Geometry: final body of the model. Coordinates: model frame, mm. A direction names the side the tool comes from. Give positions to 0.01 mm unless a question says otherwise; leave off trailing zeros. Order: outer loops, then holes, each group sorted by start corner. A loop starts at its lowest first (then second) coordinate and runs counter-clockwise, first axis right, second up. Notation, with made-up numbers: (-10.75, -35) -> (13.25, -35) arc R17 ccw to (13.25, -30) -> close; hole circle Ø7 at (83.5, 83.25). An arc over 180 degrees is marked (long way). Write item = value, one per line.
```python
from build123d import *

# Parameters (mm, degrees)
SKETCH1_R           = 1.5
BOSS_EXTRUDE1_DEPTH = 4
SKETCH1_3_R         = 3.81
SKETCH1_3_R_2       = 1.5
BOSS_EXTRUDE2_DEPTH = 7
FILLET1_R           = 30


with BuildPart() as part:
    # Sketch1 → Boss-Extrude1 (new body)
    with BuildSketch(Plane(origin=(0, 0, 0), x_dir=(1, 0, 0), z_dir=(0, 1, 0))):
        with BuildLine():
            ThreePointArc((-3.81, -46), (0, -49.81), (3.81, -46))
            Line((3.81, -46), (3.81, 46))
            ThreePointArc((3.81, 46), (2.694076836, 48.694076836), (0, 49.81))
            Line((0, 49.81), (-115.000000027, 49.81))
            ThreePointArc((-115.000000027, 49.81), (-118.81, 45.999999987), (-115, 42.19))
            Line((-115, 42.19), (-72.06, 42.19))
            Line((-72.06, 42.19), (-72.06, 17.81))
            ThreePointArc((-72.06, 17.81), (-68.25, 14), (-64.44, 17.81))
            Line((-64.44, 17.81), (-64.44, 42.19))
            Line((-64.44, 42.19), (-3.81, 42.19))
            Line((-3.81, 42.19), (-3.81, -46))
        make_face()
        with BuildLine():
            Line((-69.75, 21.62), (-69.75, 33.81))
            ThreePointArc((-69.75, 33.81), (-68.25, 35.31), (-66.75, 33.81))
            Line((-66.75, 33.81), (-66.75, 21.62))
            ThreePointArc((-66.75, 21.62), (-68.25, 20.12), (-69.75, 21.62))
        make_face(mode=Mode.SUBTRACT)
        with Locations(Location((0, -46, 0), (0, 0, 270))):
            Circle(SKETCH1_R, mode=Mode.SUBTRACT)
        with Locations(Location((0, -7.9, 0), (0, 0, 270))):
            Circle(SKETCH1_R, mode=Mode.SUBTRACT)
        with Locations(Location((0, 46, 0), (0, 0, 270))):
            Circle(SKETCH1_R, mode=Mode.SUBTRACT)
        with Locations(Location((-115, 46, 0), (0, 0, 270))):
            Circle(SKETCH1_R, mode=Mode.SUBTRACT)
    extrude(amount=BOSS_EXTRUDE1_DEPTH)

    # Sketch1_3 → Boss-Extrude2 (add)
    # profile 1 of 3: a face of its own
    with BuildSketch(Plane(origin=(0, 0, 0), x_dir=(1, 0, 0), z_dir=(0, 1, 0))):
        with Locations(Location((-115, 46, 0), (0, 0, 270))):
            Circle(SKETCH1_3_R)
        with Locations(Location((-115, 46, 0), (0, 0, 270))):
            Circle(SKETCH1_3_R_2, mode=Mode.SUBTRACT)
    # profile 2 of 3: a face of its own
    with BuildSketch(Plane(origin=(0, 0, 0), x_dir=(1, 0, 0), z_dir=(0, 1, 0))):
        with Locations(Location((0, 46, 0), (0, 0, 90))):
            Circle(SKETCH1_3_R)
        with Locations(Location((0, 46, 0), (0, 0, 270))):
            Circle(SKETCH1_3_R_2, mode=Mode.SUBTRACT)
    # profile 3 of 3: a face of its own
    with BuildSketch(Plane(origin=(0, 0, 0), x_dir=(1, 0, 0), z_dir=(0, 1, 0))):
        with Locations((0, -46)):
            Circle(SKETCH1_3_R)
        with Locations(Location((0, -46, 0), (0, 0, 270))):
            Circle(SKETCH1_3_R_2, mode=Mode.SUBTRACT)
    extrude(amount=BOSS_EXTRUDE2_DEPTH)

    # Fillet1
    fillet1_edges = [part.edges().sort_by_distance(p)[0] for p in [
        (-64.44, 2, -42.19),
        (-72.06, 2, -42.19),
        (-3.81, 2, -42.19),
    ]]
    fillet(fillet1_edges, radius=FILLET1_R)


solid = part.part
```
1) First-contact query: P1, Ø2, axis at x = -109, y = 2.5, coming from the +Z side; P2, Ø2.5, axis at x = 0, z = 46, coming from the +Y side; P3, Ø3, axis at y = 3.5, z = 1, coming from the -X side; P4, Ø3.5, axis at x = -115, z = -46, coming from the -Y side. Flat tips, straight axial feed; report the tip coordinate or a pass-through.
Check sheet entries:
P1 = -42.19
P2 = through
P3 = -3.81
P4 = 0
2) Section query D-D (x = -21.5). Output: boundary loops of the cut face in (y, z), plus the area to 3 significant figures.
Check sheet entries:
outline = (0, -49.81) -> (4, -49.81) -> (4, -39.55) -> (0, -39.55) -> close
area = 41.0 mm²
3) Section query A-A (y = 5.25). Output: boundary loops of the cut face in (x, z), plus the area to 3 significant figures.
Check sheet entries:
outline = circle Ø7.62 at (-115, -46); circle Ø7.62 at (0, -46); circle Ø7.62 at (0, 46); hole circle Ø3 at (-115, -46); hole circle Ø3 at (0, -46); hole circle Ø3 at (0, 46)
area = 116 mm²
4) Reachability of faces 4 (the face through (-47, 4, -41)), 5 (the face through (-44, 0, -41)), 6 (the face through (-68.28, 1.97, -35.31)) from +Z, -Z, +X, -X, +Y, -Y: full face, straight path, thin tool, end or side. Return the list, or none.
Check sheet entries:
face_4 = +Y
face_5 = +Z, -Z, +X, -X, -Y
face_6 = +Y, -Y
5) Section query C-C (z = 7.9). Output: boundary loops of the cut face in (x, y).
Check sheet entries:
outline = (-3.81, 0) -> (-1.5, 0) -> (-1.5, 4) -> (-3.81, 4) -> close; (1.5, 0) -> (3.81, 0) -> (3.81, 4) -> (1.5, 4) -> close
6) Line query: line 1 (X direction, y = 1.8, z = 7.9); line 2 (Z direction, x = -115, y = 4); line 3 (Z direction, x = -33.5, y = 1.75). Output: solid intervals per line, ascending. Write a range as from..to.
Check sheet entries:
line_1 = -3.81..-1.5, 1.5..3.81
line_2 = -49.81..-47.5, -44.5..-42.19
line_3 = -49.81..-42.19
7) Section query B-B (x = -68.25). Output: boundary loops of the cut face in (y, z).
Check sheet entries:
outline = (0, -49.81) -> (4, -49.81) -> (4, -35.31) -> (0, -35.31) -> close; (0, -20.12) -> (4, -20.12) -> (4, -14) -> (0, -14) -> close
8) Mould query, pull axis X, two halves, no side actions, for faces 1 (the face through (-12.365, 2.028, -33.169)), 2 (the face through (-3.81, 2, 16)), 3 (the face through (-108, 2, -42.19)). Classes: +X half, -X half, draft (parallel to the pull), parting line (faces both ways), or undercut.
Check sheet entries:
face_1 = undercut
face_2 = -X half
face_3 = draft
